Part model, mm, in its own coordinate system. A direction names the side the tool comes from. Round coordinates to 2 decimals unless told otherwise and drop trailing zeros. Write each loop counter-clockwise with the first axis right and the second up, starting at its lowest first coordinate (ties: lowest second). Pieces come first, ordered by that corner, then holes.
1) Saw through at A-A on z = -27.4. Count the separate pieces of the cut face and the enclosed holes in it, and give its area (3 significant figures).
2) Pull direction Y, two halves, no side cores. Call faces 1 (the flat face through (-1.2, 3, -3)), 2 (the cylindrical face through (1.521, -14.119, -28.926)), 3 (the flat face through (1.78, -31.79, -6.13)): +Y half, -Y half, draft (parallel to the pull), parting line (faces both ways), or undercut.
3) Drill centre lines: L1, parallel to Y at x = 2.25, z = -27.4; L2, parallel to Y at x = 2, z = -27; L3, parallel to X at y = -15, z = -14.5. Where is each one in solid material? Low to high.
4) Flat gauge pins, fed straight in: pin 1 (5 mm diameter, centred on x = -1, z = -17.5, fed in from -Y); pin 2 (2 mm diameter, centred on y = -27.5, z = -10, fed in from -X); pin 3 (5 mm diameter, centred on x = -1, z = -4.5, fed in from -Y). Where does each tip first touch, or does it go through?
5) Saw through at C-C on x = -3.5. Write the cut outline in (y, z), and give its area (3 significant figures).
6) Which spindle directions (+Z, -Z, +X, -X, +Y, -Y) get a long thin tool onto all of the face, cutting with end or side? Do faces 4 (the cylindrical face through (1.779, -6.743, -16.775)), 5 (the cylindrical face through (-4.947, 3.905, 0.867)). Say none if no direction does.
```python
from build123d import *

# Parameters (mm, degrees)
AUFSATZ_LINEAR_AUSTRAGEN1_DEPTH = 3
SKIZZE2_R                       = 4
AUFSATZ_LINEAR_AUSTRAGEN2_DEPTH = 9.1
FASE1_SIZE                      = 0.3
SKIZZE3_R                       = 1.6
SCHNITT_LINEAR_AUSTRAGEN1_DEPTH = 6
SKIZZE4_R                       = 7
AUFSATZ_LINEAR_AUSTRAGEN3_DEPTH = 1.2
VERRUNDUNG1_R                   = 1
SCHNITT_LINEAR_AUSTRAGEN2_DEPTH = 10
VERRUNDUNG3_R                   = 8
VERRUNDUNG4_R                   = 0.6
VERRUNDUNG5_R                   = 0.6


with BuildPart() as part:
    # Skizze1 → Aufsatz-Linear austragen1 (new body)
    with BuildSketch(Plane(origin=(0, 0, 0), x_dir=(0, 0, -1), z_dir=(1, 0, 0))):
        with BuildLine():
            Line((31, -11), (31, -58))
            Line((31, -58), (20.6, -58))
            Line((20.6, -58), (-8.754311744, -4.833427964))
            ThreePointArc((-8.754311744, -4.833427964), (-6.538746444, 7.566029007), (6.05088421, 7.961582774))
            Line((6.05088421, 7.961582774), (31, -11))
        make_face()
    extrude(amount=AUFSATZ_LINEAR_AUSTRAGEN1_DEPTH)

    # Skizze2 → Aufsatz-Linear austragen2 (add)
    with BuildSketch(Plane.ZY):
        with Locations(Location((0, 0, 0), (0, 0, 180))):
            Circle(SKIZZE2_R)
    extrude(amount=AUFSATZ_LINEAR_AUSTRAGEN2_DEPTH)

    # Fase1
    fase1_edges = [part.edges().sort_by_distance(p)[0] for p in [
        (-9.1, 0, 4),
    ]]
    chamfer(fase1_edges, length=FASE1_SIZE)

    # Skizze3 → Schnitt-Linear austragen1 (cut)
    with BuildSketch(Plane(origin=(3, 0, 0), x_dir=(0, 0, -1), z_dir=(1, 0, 0))):
        with Locations((27.4, -54.4)):
            Circle(SKIZZE3_R)
        with Locations((27.4, -14.6)):
            Circle(SKIZZE3_R)
    extrude(amount=-SCHNITT_LINEAR_AUSTRAGEN1_DEPTH, mode=Mode.SUBTRACT)

    # Skizze4 → Aufsatz-Linear austragen3 (add)
    with BuildSketch(Plane.ZY):
        with Locations(Location((0, 0, 0), (0, 0, 180))):
            Circle(SKIZZE4_R)
    extrude(amount=AUFSATZ_LINEAR_AUSTRAGEN3_DEPTH)

    # Verrundung1
    verrundung1_edges = [part.edges().sort_by_distance(p)[0] for p in [
        (0, 0, 7),
    ]]
    fillet(verrundung1_edges, radius=VERRUNDUNG1_R)

    # Skizze5 → Schnitt-Linear austragen2 (cut)
    with BuildSketch(Plane.ZY):
        with BuildLine():
            ThreePointArc((-31, -11), (-15.331560384, -5.721628096), (-6.05088421, 7.961582774))
            Line((-6.05088421, 7.961582774), (-31, -11))
        make_face()
    extrude(amount=-SCHNITT_LINEAR_AUSTRAGEN2_DEPTH, mode=Mode.SUBTRACT)

    # Verrundung3
    verrundung3_edges = [part.edges().sort_by_distance(p)[0] for p in [
        (1.5, 7.961582774, -6.05088421),
    ]]
    fillet(verrundung3_edges, radius=VERRUNDUNG3_R)

    # Verrundung4
    verrundung4_edges = [part.edges().sort_by_distance(p)[0] for p in [
        (0, -6.624911651, -16.597231966),
        (0, -34.5, -31),
        (0, 4.342309459, 9.008015795),
        (0, 8.970000491, -3.541995713),
        (0, -58, -25.8),
        (0, -31.416713982, -5.922844128),
    ]]
    fillet(verrundung4_edges, radius=VERRUNDUNG4_R)

    # Verrundung5
    verrundung5_edges = [part.edges().sort_by_distance(p)[0] for p in [
        (-1.2, 0, 7),
    ]]
    fillet(verrundung5_edges, radius=VERRUNDUNG5_R)


solid = part.part
```
Completed:
1. separate pieces: 3
1. enclosed holes: 0
1. area: 122 mm2
2. face 1: draft
2. face 2: undercut
2. face 3: -Y half
3. L1: y = -58 to -56, -52.8 to -16.2, -13 to -10.75
3. L2: y = -58 to -55.95, -52.85 to -16.15, -13.05 to -10.69
3. L3: x = 0 to 3
4. pin 1: stops at y = -56.09
4. pin 2: stops at x = 0
4. pin 3: stops at y = -32.54
5. outline: circle Ø8 at (0, 0)
5. area: 50.3 mm2
6. face 4: -Z, +X, -X, +Y
6. face 5: -X
